from build123d import *

# Parameters (mm, degrees)
CROQUIS1_W              = 470.5
CROQUIS1_H              = 120
CROQUIS1_R              = 1.55
SALIENTE_EXTRUIR1_DEPTH = 2
CROQUIS2_W              = 470.5
CROQUIS2_H              = 120
CROQUIS2_W_2            = 469.5
CROQUIS2_H_2            = 119
CORTAR_EXTRUIR1_DEPTH   = 2
CROQUIS3_R              = 1.6
CORTAR_EXTRUIR2_DEPTH   = 2
CROQUIS4_R              = 1.6
CROQUIS4_W              = 27
CROQUIS4_H              = 27
CORTAR_EXTRUIR3_DEPTH   = 2
REDONDEO1_R             = 2
CORTAR_EXTRUIR4_DEPTH   = 2
REDONDEO2_R             = 4
REDONDEO3_R             = 4


with BuildPart() as part:
    # Croquis1 → Saliente-Extruir1 (new body)
    with BuildSketch(Plane(origin=(0, 0, 0), x_dir=(1, 0, 0), z_dir=(0, 1, 0))):
        with Locations((235.25, 60)):
            Rectangle(CROQUIS1_W, CROQUIS1_H)
        with Locations(Location((12.5, 15, 0), (0, 0, 270))):
            Circle(CROQUIS1_R, mode=Mode.SUBTRACT)
        with Locations(Location((12.5, 110, 0), (0, 0, 270))):
            Circle(CROQUIS1_R, mode=Mode.SUBTRACT)
        with Locations(Location((458, 15, 0), (0, 0, 90))):
            Circle(CROQUIS1_R, mode=Mode.SUBTRACT)
        with Locations(Location((458, 110, 0), (0, 0, 90))):
            Circle(CROQUIS1_R, mode=Mode.SUBTRACT)
    extrude(amount=SALIENTE_EXTRUIR1_DEPTH)

    # Croquis2 → Cortar-Extruir1 (cut)
    with BuildSketch(Plane.XZ):
        with Locations((235.25, -60)):
            Rectangle(CROQUIS2_W, CROQUIS2_H)
        with Locations((235.25, -60)):
            Rectangle(CROQUIS2_W_2, CROQUIS2_H_2, mode=Mode.SUBTRACT)
    extrude(amount=-CORTAR_EXTRUIR1_DEPTH, mode=Mode.SUBTRACT)

    # Croquis3 → Cortar-Extruir2 (cut)
    with BuildSketch(Plane.XZ):
        with Locations(Location((235.25, -12.5, 0), (0, 0, 270))):
            Circle(CROQUIS3_R)
    extrude(amount=-CORTAR_EXTRUIR2_DEPTH, mode=Mode.SUBTRACT)

    # Croquis4 → Cortar-Extruir3 (cut)
    with BuildSketch(Plane.XZ):
        with Locations(Location((428.5, -66.5, 0), (0, 0, 270))):
            Circle(CROQUIS4_R)
        with Locations(Location((428.5, -13.5, 0), (0, 0, 270))):
            Circle(CROQUIS4_R)
        with Locations((428.5, -40)):
            Rectangle(CROQUIS4_W, CROQUIS4_H)
    extrude(amount=-CORTAR_EXTRUIR3_DEPTH, mode=Mode.SUBTRACT)

    # Redondeo1
    redondeo1_edges = [part.edges().sort_by_distance(p)[0] for p in [
        (415, 1, -53.5),
        (442, 1, -53.5),
        (442, 1, -26.5),
        (415, 1, -26.5),
    ]]
    fillet(redondeo1_edges, radius=REDONDEO1_R)

    # Croquis5 → Cortar-Extruir4 (cut)
    with BuildSketch(Plane.XZ):
        Polygon((25.5, -119.5), (25.5, -15.5), (220.25, -15.5), (220.25, -20.5), (250.25, -20.5), (250.25, -15.5), (400, -15.5), (400, -71.5), (445, -71.5), (445, -119.5), align=None)
    extrude(amount=-CORTAR_EXTRUIR4_DEPTH, mode=Mode.SUBTRACT)

    # Redondeo2
    redondeo2_edges = [part.edges().sort_by_distance(p)[0] for p in [
        (25.5, 1, -15.5),
        (220.25, 1, -15.5),
        (250.25, 1, -15.5),
        (400, 1, -15.5),
        (400, 1, -71.5),
        (445, 1, -71.5),
    ]]
    fillet(redondeo2_edges, radius=REDONDEO2_R)

    # Redondeo3
    redondeo3_edges = [part.edges().sort_by_distance(p)[0] for p in [
        (220.25, 1, -20.5),
        (250.25, 1, -20.5),
    ]]
    fillet(redondeo3_edges, radius=REDONDEO3_R)


solid = part.part
Build history of the part. All positions in model axes, mm. Round coordinates to 2 decimals unless told otherwise and drop trailing zeros. Loops run counter-clockwise (first coordinate to the right, second up) from the corner with the lowest first, then second, coordinate; pieces in that order, holes last. Notation, with made-up numbers: (62, 66) -> (110, 66) arc R18 ccw to (110, 91) -> close; hole circle Ø7 at (43.5, 19). An arc over 180 degrees is marked (long way). Answer in a Markdown table with one row per item.
Item 1: Saw through at B-B (x = 371). Write the cut outline in (y, z), and give its area (3 significant figures).
Answers below:
| item | result |
|---|---|
| outline | (0, -15.5) -> (2, -15.5) -> (2, -0.5) -> (0, -0.5) -> close |
| area | 30.0 mm² |
Item 2: Saw through at A-A (z = -100). Write the cut outline in (x, y), and give its area (3 significant figures).
Answers below:
| item | result |
|---|---|
| outline | (0.5, 0) -> (25.5, 0) -> (25.5, 2) -> (0.5, 2) -> close; (445, 0) -> (470, 0) -> (470, 2) -> (445, 2) -> close |
| area | 100 mm² |
Item 3: Pin check, flat tips, straight feed: pin 1 (3.5 mm diameter, centred on x = 235.25, z = -12.5, fed in from -Y); pin 2 (2.5 mm diameter, centred on x = 458, z = -15, fed in from -Y); pin 3 (0.6 mm diameter, centred on x = 164, y = 0.5, fed in from -Z). Stop position of each tip, or through.
Answers below:
| item | result |
|---|---|
| pin 1 | stops at y = 0 |
| pin 2 | passes through |
| pin 3 | stops at z = -15.5 |
Item 4: Saw through at C-C (y = 1.35). State how many separate pieces and enclosed holes the cut face has, and give its area (3 significant figures).
Answers below:
| item | result |
|---|---|
| separate pieces | 1 |
| enclosed holes | 8 |
| area | 14,100 mm² |
Item 5: Drill centre lines: L1, parallel to Z at x = 428.5, y = 0.9; L2, parallel to X at y = 0.4, z = -110; L3, parallel to X at y = 1.5, z = -98.5. Where is each one in solid material? Low to high. Write a range as [from, to].
Answers below:
| item | result |
|---|---|
| L1 | z = [-71.5, -68.1], [-64.9, -53.5], [-26.5, -15.1], [-11.9, -0.5] |
| L2 | x = [0.5, 10.95], [14.05, 25.5], [445, 456.45], [459.55, 470] |
| L3 | x = [0.5, 25.5], [445, 470] |
